Design review of the part built by this model. Coordinates are the model's own, in mm. A direction names the side the tool comes from. Give positions to 0.01 mm unless a question says otherwise; leave off trailing zeros. Loops run counter-clockwise (first coordinate to the right, second up) from the corner with the lowest first, then second, coordinate; pieces in that order, holes last. Notation, with made-up numbers: (24, 62) - (29, 62) arc R14 ccw to (29, 81) - close; hole circle Ø8 at (87, -15). An arc over 180 degrees is marked (long way). One line per item, written item: value. Start each with the question number.
```python
from build123d import *

# Parameters (mm, degrees)
BOSS_EXTRUDE1_DEPTH     = 2
SKETCH2_W               = 8.5
SKETCH2_H               = 8
BOSS_EXTRUDE2_DEPTH     = 6
SKETCH3_R               = 3.5
BOSS_EXTRUDE3_DEPTH     = 2
FILLET1_R               = 1
SKETCH4_R               = 25.5
BOSS_EXTRUDE4_DEPTH     = 21
FILLET2_R               = 3
SKETCH6_W               = 16
SKETCH6_H               = 16
BOSS_EXTRUDE5_DEPTH     = 16
CUT_EXTRUDE1_DEPTH      = 66.3471499
CUT_EXTRUDE1_DEPTH_BACK = 66.3471499
SKETCH7_R               = 1.75


with BuildPart() as part:
    # Sketch1 → Boss-Extrude1 (new body)
    with BuildSketch(Plane.XY):
        with BuildLine():
            Line((44.5, 36), (37.5, 43))
            Line((37.5, 43), (22, 43))
            Line((22, 43), (19.5, 40.5))
            Line((19.5, 40.5), (-19.5, 40.5))
            Line((-19.5, 40.5), (-22, 43))
            Line((-22, 43), (-37.5, 43))
            Line((-37.5, 43), (-44.5, 36))
            Line((-44.5, 36), (-44.5, 1.5))
            ThreePointArc((-44.5, 1.5), (-40, -3), (-44.5, -7.5))
            Line((-44.5, -7.5), (-44.5, -36))
            Line((-44.5, -36), (-37.5, -43))
            Line((-37.5, -43), (37.5, -43))
            Line((37.5, -43), (44.5, -36))
            Line((44.5, -36), (44.5, -7.5))
            ThreePointArc((44.5, -7.5), (40, -3), (44.5, 1.5))
            Line((44.5, 1.5), (44.5, 36))
        make_face()
    extrude(amount=-BOSS_EXTRUDE1_DEPTH)

    # Sketch2 → Boss-Extrude2 (add)
    with BuildSketch(Plane.XY):
        with Locations((-39.25, 32)):
            Rectangle(SKETCH2_W, SKETCH2_H)
        with Locations((38.75, 32)):
            Rectangle(SKETCH2_W, SKETCH2_H)
        with Locations((38.75, 15)):
            Rectangle(SKETCH2_W, SKETCH2_H)
        with Locations((-39.25, 15)):
            Rectangle(SKETCH2_W, SKETCH2_H)
    extrude(amount=BOSS_EXTRUDE2_DEPTH)

    # Sketch3 → Boss-Extrude3 (add)
    with BuildSketch(Plane.XY.offset(6)):
        with Locations((-39.25, 32)):
            Circle(SKETCH3_R)
        with Locations((38.75, 32)):
            Circle(SKETCH3_R)
        with Locations((38.75, 15)):
            Circle(SKETCH3_R)
        with Locations((-39.25, 15)):
            Circle(SKETCH3_R)
    extrude(amount=BOSS_EXTRUDE3_DEPTH)

    # Fillet1
    fillet1_edges = [part.edges().sort_by_distance(p)[0] for p in [
        (35.25, 32, 8),
        (35.25, 15, 8),
        (-42.75, 15, 8),
        (-42.75, 32, 8),
    ]]
    fillet(fillet1_edges, radius=FILLET1_R)

    # Sketch4 → Boss-Extrude4 (add)
    with BuildSketch(Plane.XY):
        with Locations(Location((0, 15, 0), (0, 0, 90))):
            Circle(SKETCH4_R)
    extrude(amount=BOSS_EXTRUDE4_DEPTH)

    # Fillet2
    fillet2_edges = [part.edges().sort_by_distance(p)[0] for p in [
        (0, -10.5, 21),
    ]]
    fillet(fillet2_edges, radius=FILLET2_R)

    # Sketch6 → Boss-Extrude5 (add)
    with BuildSketch(Plane.XY):
        with Locations((20.355257786, -28.630901536)):
            Rectangle(SKETCH6_W, SKETCH6_H)
        with Locations((-22.644742214, -28.630901536)):
            Rectangle(SKETCH6_W, SKETCH6_H)
    extrude(amount=BOSS_EXTRUDE5_DEPTH)

    # Sketch7 → Cut-Extrude1 (cut, two sides: drawn at the far end of the back side and taken through both)
    with BuildSketch(Plane.XY.offset(-CUT_EXTRUDE1_DEPTH_BACK)):
        with Locations((-27.5, 36.5)):
            Circle(SKETCH7_R)
        with Locations((27.5, 36.5)):
            Circle(SKETCH7_R)
        with Locations((-38, -36.5)):
            Circle(SKETCH7_R)
        with Locations((38.5, -36.5)):
            Circle(SKETCH7_R)
    extrude(amount=CUT_EXTRUDE1_DEPTH + CUT_EXTRUDE1_DEPTH_BACK, mode=Mode.SUBTRACT)


solid = part.part
```
(1) To check wall thickness, follow L1, parallel to Y at x = 27.5, z = -1.3; L2, parallel to X at y = -34, z = 3; L3, parallel to X at y = -36.5, z = -0.6. State the ranges of each line that lie inside material, in increasing order. Write a range as from..to.
(2) Machinability: for faces 1 (the flat face through (43, 32, 3)), 2 (the flat face through (-23, -20.631, 8)), 3 (the flat face through (-21, 42, -1)), 4 (the flat face through (-40.3, 11.5, 6)), which of the approach directions +Z, -Z, +X, -X, +Y, -Y give a long, thin tool a straight path to every point of the face, cutting with its end or side? Answer none if there is none.
(3) Take a section at A-A on x = -27.5. State the section outline as (y, z) points.
(4) For pin 1 Ø6 at (y, z) = (6, 7.5) entering from +X; pin 2 Ø2 at (x, z) = (-30.5, 9.5) entering from +Y; pin 3 Ø4.5 at (x, y) = (38.5, -36.5) entering from +Z, all flat-tipped, find the tip position at first contact; note any pin that passes through.
(5) Draft analysis for pull direction Y (two halves, no side actions). For faces 5 (the cylindrical face through (40, -3, -1)), 6 (the flat face through (-35, 15, 3)), 7 (the cylindrical face through (36.2, 34.4, 6.5)), 8 (the flat face through (39, 11, 3)), state which applies: pulls with the +Y half, pulls with the -Y half, needs draft (parallel to the pull), parting line crosses it, or undercut.
Here are the results:
1. L1: -43..34.75, 38.25..43
1. L2: -30.64..-14.64, 12.36..28.36
1. L3: -44..-39.75, -36.25..36.75, 40.25..44
2. face 1: +Z, +X, +Y, -Y
2. face 2: +Z, +X, -X
2. face 3: +Z, -Z, +Y
2. face 4: +Z
3. outline: (-43, -2) - (34.75, -2) - (34.75, 0) - (-20.63, 0) - (-20.63, 16) - (-36.63, 16) - (-36.63, 0) - (-43, 0) - close; (38.25, -2) - (43, -2) - (43, 0) - (38.25, 0) - close
4. pin 1: x = 24.78
4. pin 2: y = -20.63
4. pin 3: z = 0
5. face 5: undercut
5. face 6: needs draft
5. face 7: undercut
5. face 8: pulls with the -Y half
